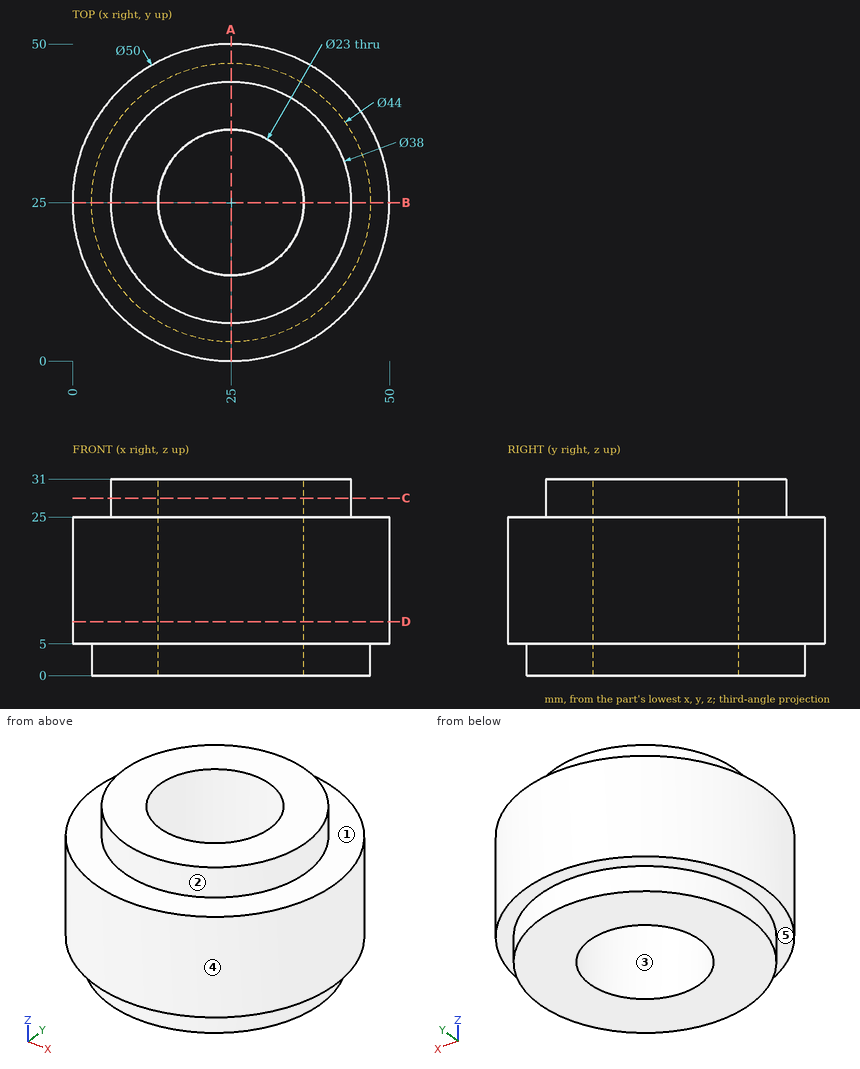
Verification items for this drawing (mm, ordinates from the low corner). A direction names the side the tool comes from. Give positions to 0.01 mm unless a question says otherwise; leave off trailing zeros. Loops run counter-clockwise (first coordinate to the right, second up) from the corner with the lowest first, then second, coordinate; pieces in that order, holes last. Notation, with made-up numbers: M 17.5,56.25 L 23.5,56.25 A32 cw 23.5,91.25 Z; hole C 3,46.25 d10. An arc over 180 degrees is marked long. Return JSON: item names as keys, results as strings. Group by question number.
1. Mould release check, pull along Y, two halves, no side actions. Record for the marked faces 1, 2 and 3: released by +Y, released by -Y, zero draft, split by the parting line, or undercut.
2. Thickness scan on L1, parallel to Y at x = 25, z = 15; L2, parallel to Z at x = 48, y = 16; L3, parallel to Y at x = 19, z = 21.5. Record the ranges inside material, lowest first.
3. Cross-section at A-A on x = 25. Record the boundary of the cut face in (y, z).
4. Go/stop test with flat-tipped pins: pin 1 (8 mm diameter, centred on x = 28.5, z = 19, fed in from -Y); pin 2 (1 mm diameter, centred on y = 18, z = 22, fed in from -X); pin 3 (1.5 mm diameter, centred on y = 38, z = 3.5, fed in from +X). Record where each tip stops, or that it passes through.
5. Cross-section at C-C on z = 28. Record the boundary of the cut face in (x, y).
6. Tool access check on the marked faces 4 and 5. Record the directions out of +Z, -Z, +X, -X, +Y, -Y that give a thin tool (end or side, any length) a straight path to the whole face; none if there is none.
7. Cross-section at D-D on z = 8.5. Record the boundary of the cut face in (x, y).
Return value:
{
 "1": {"face 1": "zero draft", "face 2": "split by the parting line", "face 3": "undercut"},
 "2": {"L1": "0 to 13.5, 36.5 to 50", "L2": "5 to 25", "L3": "0.73 to 15.19, 34.81 to 49.27"},
 "3": {"outline": "M 0,5 L 3,5 L 3,0 L 13.5,0 L 13.5,31 L 6,31 L 6,25 L 0,25 Z; M 36.5,0 L 47,0 L 47,5 L 50,5 L 50,25 L 44,25 L 44,31 L 36.5,31 Z"},
 "4": {"pin 1": "y = 0", "pin 2": "x = 0.86", "pin 3": "x = 43.27"},
 "5": {"outline": "C 25,25 d38; hole C 25,25 d23"},
 "6": {"face 4": "+Z, -Z", "face 5": "-Z"},
 "7": {"outline": "C 25,25 d50; hole C 25,25 d23"}
}
